Here's the drawing with two shaded views (mm, measured from the low corner). I have some questions. Coordinates: 2 decimals unless noted, no trailing zeros. Loops run counter-clockwise (first coordinate to the right, second up) from the corner with the lowest first, then second, coordinate; pieces in that order, holes last.
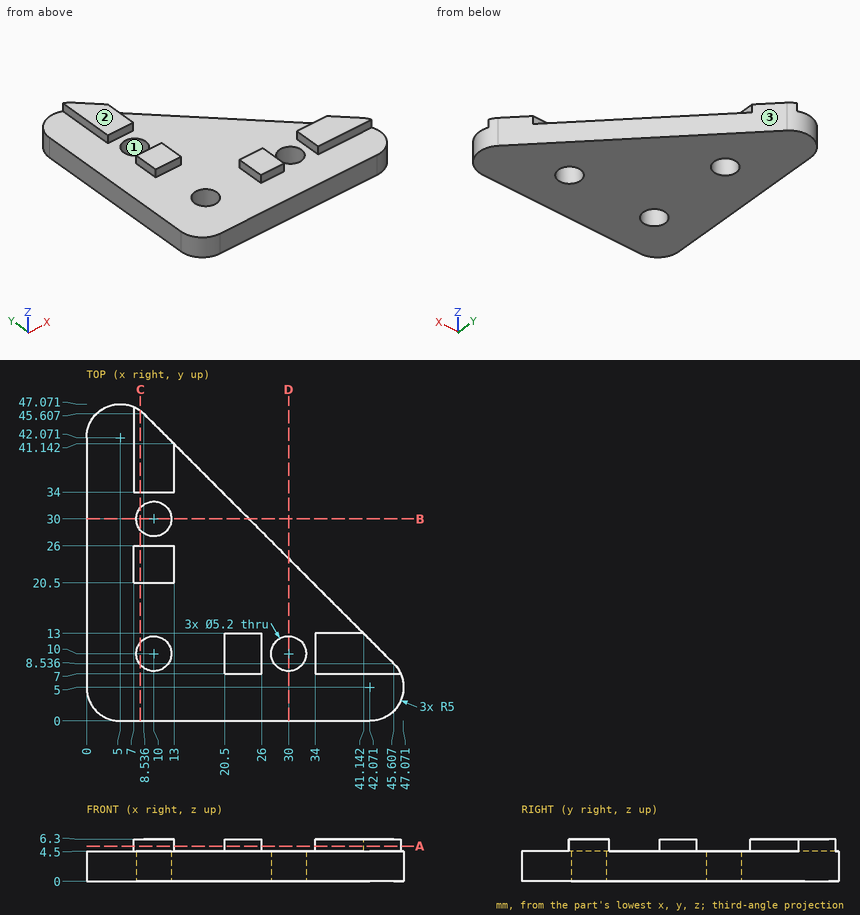
(1) I'm going to push flat-ended pins straight in: pin 1 (0.5 mm diameter, centred on x = 10.5, z = 6, fed in from +Y); pin 2 (0.9 mm diameter, centred on y = 36.5, z = 5, fed in from +X); pin 3 (2 mm diameter, centred on x = 14.5, z = 2, fed in from +Y). Where does each tip first touch, or does it pass through?
Check values:
pin 1: stops at y = 43.89
pin 2: stops at x = 13
pin 3: stops at y = 40.64
(2) I want a section at B-B on y = 30. Write out the boundary of the cut face in (x, z).
Check values:
outline: (0, 0) - (7.4, 0) - (7.4, 4.5) - (0, 4.5) - close; (12.6, 0) - (24.14, 0) - (24.14, 4.5) - (12.6, 4.5) - close
(3) If we mould it in two halves opening along X, with no side actions, what happens to the marked faces 1, 2 and 3? For each: released by +X, released by -X, zero draft, split by the parting line, or undercut.
Check values:
face 1: undercut
face 2: zero draft
face 3: released by +X
(4) If I drill on probe 1 along Y at (x, z) = (10, 2.4); probe 2 along Y at (x, z) = (13, 3); probe 3 along Z at (x, y) = (25.5, 24.5), over which ranges is the centre line in solid material (lowest first)?
Check values:
probe 1: y = 0 to 7.4, 12.6 to 27.4, 32.6 to 44.14
probe 2: y = 0 to 41.14
probe 3: z = 0 to 4.5
(5) I want a section at C-C on x = 8. Write out the boundary of the cut face in (y, z), then the cut area to 3 significant figures.
Check values:
outline: (0, 0) - (8.34, 0) - (8.34, 4.5) - (0, 4.5) - close; (11.66, 0) - (28.34, 0) - (28.34, 4.5) - (26, 4.5) - (26, 6.3) - (20.5, 6.3) - (20.5, 4.5) - (11.66, 4.5) - close; (31.66, 0) - (46.07, 0) - (46.07, 6.3) - (34, 6.3) - (34, 4.5) - (31.66, 4.5) - close
area: 209 mm2
(6) I want a section at A-A on z = 5.25. Write out the boundary of the cut face in (x, y) (1 decimal), then the cut area to 3 significant figures.
Check values:
outline: (7, 20.5) - (13, 20.5) - (13, 26) - (7, 26) - close; (7, 34) - (13, 34) - (13, 41.1) - (8.5, 45.6) arc R5 ccw to (7, 46.7) - close; (20.5, 7) - (26, 7) - (26, 13) - (20.5, 13) - close; (34, 7) - (46.7, 7) arc R5 ccw to (45.6, 8.5) - (41.1, 13) - (34, 13) - close
area: 187 mm2
